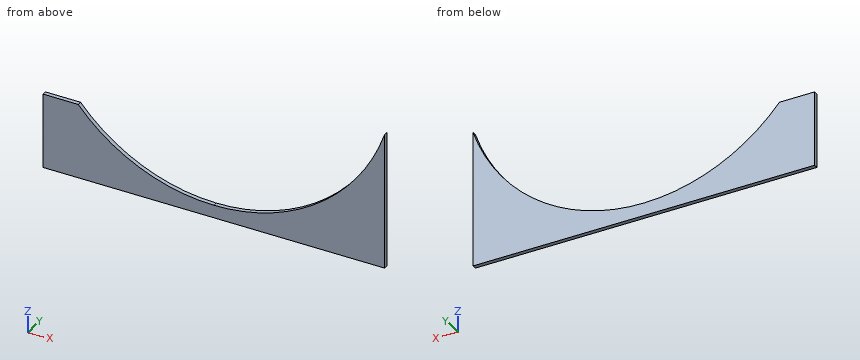
```python
from build123d import *

# Parameters (mm, degrees)
BOSS_EXTRUDE1_DEPTH = 6.35
CUT_EXTRUDE1_DEPTH  = 328.825476626


with BuildPart() as part:
    # Sketch1 → Boss-Extrude1 (new body)
    with BuildSketch(Plane(origin=(0, 0, 0), x_dir=(1, 0, 0), z_dir=(0, 1, 0))):
        with BuildLine():
            Line((257.175, 0), (-257.175, 0))
            Line((-257.175, 0), (-257.175, -203.2))
            ThreePointArc((-257.175, -203.2), (-158.153567084, -69.834458038), (0, -19.05))
            ThreePointArc((0, -19.05), (158.153567084, -69.834458038), (257.175, -203.2))
            Line((257.175, -203.2), (257.175, 0))
        make_face()
    extrude(amount=BOSS_EXTRUDE1_DEPTH)

    # Sketch2 → Cut-Extrude1 (cut, through all)
    with BuildSketch(Plane(origin=(0, 6.35, 0), x_dir=(1, 0, 0), z_dir=(0, 1, 0))):
        with BuildLine():
            Line((-257.175, -111.6203), (-204.266839371, -111.6203))
            ThreePointArc((-204.266839371, -111.6203), (-235.22086035, -154.810408098), (-257.175, -203.2))
            Line((-257.175, -203.2), (-257.175, -111.6203))
        make_face()
    extrude(amount=-CUT_EXTRUDE1_DEPTH, mode=Mode.SUBTRACT)


solid = part.part
```
CAD build for the part. Positions are in the model's coordinates, mm. Round coordinates to 2 decimals unless told otherwise and drop trailing zeros. Write each loop counter-clockwise with the first axis right and the second up, starting at its lowest first coordinate (ties: lowest second). Pieces come first, ordered by that corner, then holes.
Item 1: Drill centre lines: L1, parallel to X at y = 2.25, z = 66 (3 decimals); L2, parallel to X at y = 1.25, z = 79.5 (3 decimals); L3, parallel to X at y = 4.25, z = 116 (3 decimals). Where is each one in solid material? Low to high.
Filled in:
L1: x = -257.175 to -152.657, 152.657 to 257.175
L2: x = -257.175 to -170.847, 170.847 to 257.175
L3: x = 208.025 to 257.175
Item 2: Band-saw the part on A-A on z = 58. Write the cut outline in (x, y) (3 decimals).
Filled in:
outline: (-257.175, 0) - (-140.16, 0) - (-140.16, 6.35) - (-257.175, 6.35) - close; (140.16, 0) - (257.175, 0) - (257.175, 6.35) - (140.16, 6.35) - close
Item 3: Band-saw the part on C-C on x = -218.5. Write the cut outline in (y, z).
Filled in:
outline: (0, 0) - (6.35, 0) - (6.35, 111.62) - (0, 111.62) - close
Item 4: Band-saw the part on D-D on z = 94. Write the cut outline in (x, y) (3 decimals), then the cut area to 3 significant figures.
Filled in:
outline: (-257.175, 0) - (-187.359, 0) - (-187.359, 6.35) - (-257.175, 6.35) - close; (187.359, 0) - (257.175, 0) - (257.175, 6.35) - (187.359, 6.35) - close
area: 887 mm2
Item 5: Band-saw the part on B-B on y = 4. Write the cut outline in (x, z) (3 decimals).
Filled in:
outline: (-257.175, 0) - (257.175, 0) - (257.175, 203.2) arc R271.654 cw to (-204.267, 111.62) - (-257.175, 111.62) - close
